from build123d import *

# Parameters (mm, degrees)
F1_DEPTH = 101.6
F2_W     = 25.4
F2_H     = 101.6
F3_DEPTH = 50.8
F4_W     = 152.4
F4_H     = 31.2542108059
F5_DEPTH = 50.8
F6_W     = 50.8
F6_H     = 76.2
F7_DEPTH = 50.8


with BuildPart() as f1:
    # F0 (on Front) → F1 (new body)
    with BuildSketch(Plane.XZ):
        Polygon((0, 37.7466529608), (-76.2, 37.7466529608), (-76.2, -63.8533470392), (127, -63.8533470392), (127, -13.0533470392), (0, -13.0533470392), align=None)
    extrude(amount=F1_DEPTH)

    # F2 (on face) → F3 (cut)
    with BuildSketch(Plane.XY.offset(-13.0533470392)):
        with Locations((-12.7, -50.8)):
            Rectangle(F2_W, F2_H)
    extrude(amount=F3_DEPTH, mode=Mode.SUBTRACT)

    # F4 (on face) → F5 (cut)
    with BuildSketch(Plane.XY.offset(-13.0533470392)):
        with Locations((50.8, -85.9728945971)):
            Rectangle(F4_W, F4_H)
    extrude(amount=-F5_DEPTH, mode=Mode.SUBTRACT)

    # F6 (on face) → F7 (cut)
    with BuildSketch(Plane.XY.offset(37.7466529608)):
        with Locations((-50.8, -63.5)):
            Rectangle(F6_W, F6_H)
    extrude(amount=-F7_DEPTH, mode=Mode.SUBTRACT)


solid = f1.part
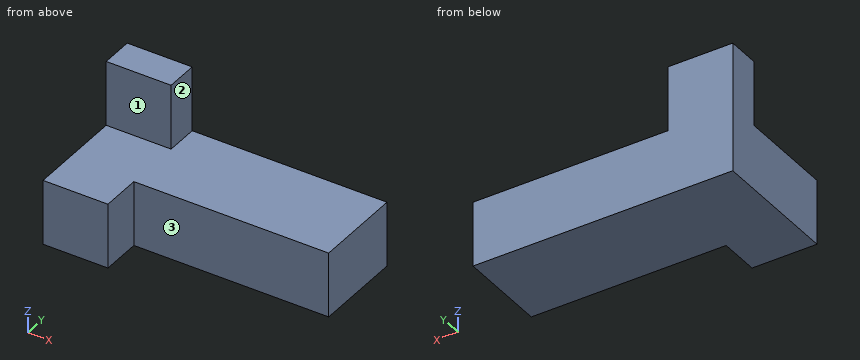
Source: CAD feature listing. Evaluate the final solid. Frame: model axes, mm. Face numbers are marked on the shaded views. A direction names the side the tool comes from. Round coordinates to 2 decimals unless told otherwise and drop trailing zeros. Loops run counter-clockwise (first coordinate to the right, second up) from the corner with the lowest first, then second, coordinate; pieces in that order, holes last. Notation, with made-up numbers: (-7, 20.25) - (30, 20.25) arc R14 cw to (30, 47.25) - close; hole circle Ø2 at (5, 39). An arc over 180 degrees is marked (long way). Write item = value, one per line. Start each with the question number.
Item 1: Reachability of the marked faces 1, 2 and 3 from +Z, -Z, +X, -X, +Y, -Y: full face, straight path, thin tool, end or side. Return the list, or none.
Item 2: First-contact query: pin 1 Ø2 at (x, z) = (-28, -49) entering from +Y; pin 2 Ø15 at (x, z) = (22, -31.5) entering from -Y; pin 3 Ø5 at (x, y) = (-34.5, -48.5) entering from +Z; pin 4 Ø20.5 at (y, z) = (-12, 1.5) entering from +X. Flat tips, straight axial feed; report the tip coordinate or a pass-through.
Item 3: Section query D-D on z = -10. Output: boundary loops of the cut face in (x, y).
Item 4: Section query B-B on z = -49. Output: boundary loops of the cut face in (x, y), plus the area to 3 significant figures.
Item 5: Material intervals for line 1 (X direction, y = -96.5, z = -31); line 2 (Y direction, x = -43, z = 8.5); line 3 (Y direction, x = 29, z = -13.5), sorted ascending.
Item 6: Section query A-A on y = -22. Output: boundary loops of the cut face in (x, z), plus the area to 3 significant figures.
Item 7: Section query C-C on x = -22. Output: boundary loops of the cut face in (y, z).
Results list:
q1.face_1 = +Z, +X, -X, -Y
q1.face_2 = +Z, +X, +Y, -Y
q1.face_3 = +Z, -Z, +X, -Y
q2.pin_1 = 0
q2.pin_2 = -70.35
q2.pin_3 = -13.05
q2.pin_4 = -25.4
q3.outline = (-76.2, -25.4) - (-25.4, -25.4) - (-25.4, 0) - (-76.2, 0) - close
q4.outline = (-76.2, -101.6) - (-25.4, -101.6) - (-25.4, -70.35) - (127, -70.35) - (127, 0) - (-76.2, 0) - close
q4.area = 15,900 mm²
q5.line_1 = -76.2 to -25.4
q5.line_2 = -25.4 to 0
q5.line_3 = -70.35 to 0
q6.outline = (-76.2, -63.85) - (127, -63.85) - (127, -13.05) - (-25.4, -13.05) - (-25.4, 37.75) - (-76.2, 37.75) - close
q6.area = 12,900 mm²
q7.outline = (-70.35, -63.85) - (0, -63.85) - (0, -13.05) - (-70.35, -13.05) - close
